```python
from build123d import *

# Parameters (mm, degrees)
BOSS_EXTRUDE2_DEPTH     = 40
SKETCH2_W               = 10
SKETCH2_H               = 40
BOSS_EXTRUDE3_DEPTH     = 20
CUT_EXTRUDE1_DEPTH      = 20
CUT_EXTRUDE1_DEPTH_BACK = 20
CUT_EXTRUDE4_DEPTH      = 51


with BuildPart() as part:
    # Sketch1 → Boss-Extrude2 (new body)
    with BuildSketch(Plane.XY):
        with BuildLine():
            ThreePointArc((20, 0), (0, 20), (-20, 0))
            Line((-20, 0), (-10, 0))
            ThreePointArc((-10, 0), (0, 10), (10, 0))
            Line((10, 0), (20, 0))
        make_face()
    extrude(amount=BOSS_EXTRUDE2_DEPTH)

    # Sketch2 → Boss-Extrude3 (add)
    with BuildSketch(Plane.XZ):
        with Locations((-15, 20)):
            Rectangle(SKETCH2_W, SKETCH2_H)
        with Locations((15, 20)):
            Rectangle(SKETCH2_W, SKETCH2_H)
    extrude(amount=BOSS_EXTRUDE3_DEPTH)

    # Sketch3 → Cut-Extrude1 (cut, two sides)
    with BuildSketch(Plane(origin=(0, 0, 0), x_dir=(1, 0, 0), z_dir=(0, 1, 0))) as cut_extrude1_sk:
        with BuildLine():
            ThreePointArc((0, -40), (-14.142135624, -34.142135624), (-20, -20))
            Line((-20, -20), (-20, -40))
            Line((-20, -40), (0, -40))
        make_face()
        with BuildLine():
            ThreePointArc((20, -20), (14.142135624, -34.142135624), (0, -40))
            Line((0, -40), (20, -40))
            Line((20, -40), (20, -20))
        make_face()
    extrude(amount=CUT_EXTRUDE1_DEPTH, mode=Mode.SUBTRACT)
    extrude(cut_extrude1_sk.sketch, amount=-CUT_EXTRUDE1_DEPTH_BACK, mode=Mode.SUBTRACT)

    # Sketch6 → Cut-Extrude4 (cut)
    with BuildSketch(Plane(origin=(0, 11, 0), x_dir=(1, 0, 0), z_dir=(0, 1, 0))):
        with BuildLine():
            Line((-10, -20), (-10, 0))
            Line((-10, 0), (10, 0))
            Line((10, 0), (10, -20))
            ThreePointArc((10, -20), (0, -30), (-10, -20))
        make_face()
    extrude(amount=CUT_EXTRUDE4_DEPTH, mode=Mode.SUBTRACT)


solid = part.part
```
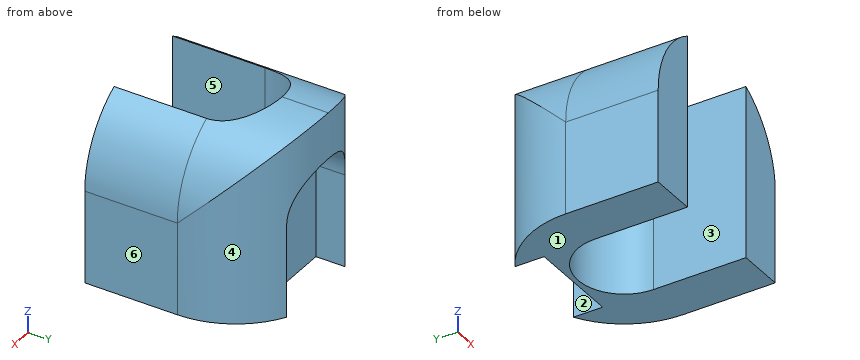
The listing builds one solid part. Answer for the finished solid, in the listing's coordinates (mm). Face numbers are marked on the shaded views. A direction names the side the tool comes from. Give positions to 0.01 mm unless a question says otherwise; leave off trailing zeros. Loops run counter-clockwise (first coordinate to the right, second up) from the corner with the lowest first, then second, coordinate; pieces in that order, holes last. Notation, with made-up numbers: (10.5, 43.25) - (16.5, 43.25) arc R21 ccw to (16.5, 78.25) - close; hole circle Ø4 at (40.25, 58). An arc over 180 degrees is marked (long way). Return JSON: item names as keys, results as strings. Group by question number.
1. Find section A-A (y = -3.5). Write down the section's boundary in (x, z), then the cut area to 3 significant figures.
2. Find section D-D (y = 14). Write down the section's boundary in (x, z).
3. Which of the six approach directions +Z, -Z, +X, -X, +Y, -Y give full straight-line access (tool end or side, diameter ignored) to the marked faces 1, 2 and 3?
4. Find section B-B (z = 6). Write down the section's boundary in (x, y).
5. Determine the mould class of the marked faces 4, 5 and 6 for opening direction X: pulls with the +X half, pulls with the -X half, needs draft (parallel to the pull), parting line crosses it, or undercut.
6. Find section C-C (x = 12). Write down the section's boundary in (y, z).
7. Given pin 1 Ø3 at (x, y) = (-7, 15) entering from -Z; pin 2 Ø5 at (y, z) = (-6.5, 34.5) entering from +X; pin 3 Ø5 at (y, z) = (15.5, 9) entering from -X, each flat-ended and moving along its own axis, determine where each tip first touches the part or whether it passes through.
8. Straight lines are drawn through the part: line 1 (X direction, y = -0.5, z = 8.5); line 2 (X direction, y = -7.5, z = 23); line 3 (Y direction, x = 9, z = 28.5). For each, find the intervals that lie inside material, in ascending order. Write a range as [from, to].
Verdict:
{
 "1": {"outline": "(-20, 0) - (-10, 0) - (-10, 37.32) arc R20 ccw to (-20, 20) - close; (10, 0) - (20, 0) - (20, 20) arc R20 ccw to (10, 37.32) - close", "area": "646 mm^2"},
 "2": {"outline": "(-14.28, 0) - (-10, 0) - (-10, 20) arc R10 cw to (10, 20) - (10, 0) - (14.28, 0) - (14.28, 34) arc R20 ccw to (-14.28, 34) - close"},
 "3": {"face 1": "-Z, +X, -X, +Y, -Y", "face 2": "-Z, +Y", "face 3": "+Z, -Z, -Y"},
 "4": {"outline": "(-20, -20) - (-10, -20) - (-10, 0) arc R10 cw to (10, 0) - (10, -20) - (20, -20) - (20, 0) arc R20 ccw to (10, 17.32) - (10, 11) - (-10, 11) - (-10, 17.32) arc R20 ccw to (-20, 0) - close"},
 "5": {"face 4": "parting line crosses it", "face 5": "undercut", "face 6": "pulls with the +X half"},
 "6": {"outline": "(-20, 0) - (16, 0) - (16, 36) - (-20, 36) - close"},
 "7": {"pin 1": "stops at z = 25.27", "pin 2": "stops at x = 16", "pin 3": "stops at x = -15.2"},
 "8": {"line 1": "x = [-20, -10], [10, 20]", "line 2": "x = [-19.77, -10], [10, 19.77]", "line 3": "y = [4.36, 17.86]"}
}
